Design review of the part built by this model. Coordinates are the model's own, in mm. Round coordinates to 2 decimals unless told otherwise and drop trailing zeros. Loops run counter-clockwise (first coordinate to the right, second up) from the corner with the lowest first, then second, coordinate; pieces in that order, holes last. Notation, with made-up numbers: (12.5, 12.25) - (55.5, 12.25) arc R16 ccw to (55.5, 40.25) - close; hole circle Ø7 at (-34, 20). An arc over 180 degrees is marked (long way). Return JSON: item names as keys, results as strings. Group by question number.
(1) We need section B-B, the plane y = 10.1. Write out the cut boundary in (x, z), and give its area (3 significant figures).
(2) Clearance check with flat-ended pins moving along their axes: pin 1 (0.5 mm diameter, centred on y = 10, z = 35, fed in from -X); pin 2 (0.5 mm diameter, centred on y = 10, z = 56.5, fed in from +X); pin 3 (1.7 mm diameter, centred on x = -9, z = 23.5, fed in from -Y); pin 4 (1.5 mm diameter, centred on x = -11, y = 12, fed in from -Z). State where each tip first meets the part, or that it passes through.
(3) We need section A-A, the plane z = 42. Write out the cut boundary in (x, y), and give its area (3 significant figures).
(4) Wall thickness on L1, parallel to X at y = 12.65, z = 52.5; L2, parallel to Y at x = -9.4, z = 38.5; L3, parallel to Y at x = -11.1, z = 28.5: over which ranges is each line inside the solid? List them lowest first. Write a range as [from, to].
(5) We need section C-C, the plane x = -9.35. Write out the cut boundary in (y, z).
from build123d import *

# Parameters (mm, degrees)
F1_DEPTH = 82.55


with BuildPart() as f1:
    # F0 (on Top) → F1 (new body)
    with BuildSketch(Plane.XY):
        with BuildLine():
            Line((-11.57952, 10.962582), (-11.57952, 9.384583))
            ThreePointArc((-11.57952, 9.384583), (-10.88102, 9.279832), (-10.18252, 9.384583))
            Line((-10.18252, 9.384583), (-10.18252, 10.962582))
            Line((-10.18252, 10.962582), (-8.604521, 10.962582))
            ThreePointArc((-8.604521, 10.962582), (-8.49977, 11.661082), (-8.604521, 12.359582))
            Line((-8.604521, 12.359582), (-10.18252, 12.359582))
            Line((-10.18252, 12.359582), (-10.18252, 13.937582))
            ThreePointArc((-10.18252, 13.937582), (-10.88102, 14.042332), (-11.57952, 13.937582))
            Line((-11.57952, 13.937582), (-11.57952, 12.359582))
            Line((-11.57952, 12.359582), (-13.157519, 12.359582))
            ThreePointArc((-13.157519, 12.359582), (-13.26227, 11.661082), (-13.157519, 10.962582))
            Line((-13.157519, 10.962582), (-11.57952, 10.962582))
        make_face()
    extrude(amount=F1_DEPTH)


solid = f1.part
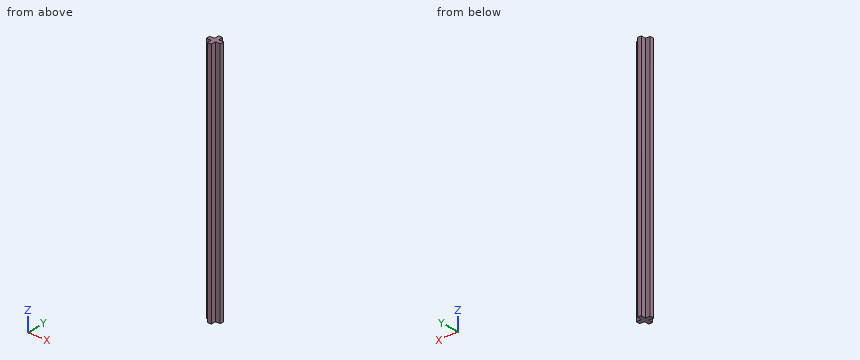
Solutions:
{
 "1": {"outline": "(-11.58, 0) - (-10.18, 0) - (-10.18, 82.55) - (-11.58, 82.55) - close", "area": "115 mm^2"},
 "2": {"pin 1": "x = -11.58", "pin 2": "x = -10.18", "pin 3": "y = 10.96", "pin 4": "z = 0"},
 "3": {"outline": "(-13.16, 10.96) - (-11.58, 10.96) - (-11.58, 9.38) arc R2.38 ccw to (-10.18, 9.38) - (-10.18, 10.96) - (-8.6, 10.96) arc R2.38 ccw to (-8.6, 12.36) - (-10.18, 12.36) - (-10.18, 13.94) arc R2.38 ccw to (-11.58, 13.94) - (-11.58, 12.36) - (-13.16, 12.36) arc R2.38 ccw to start", "area": "11.2 mm^2"},
 "4": {"L1": "[-11.58, -10.18]", "L2": "[10.96, 12.36]", "L3": "[9.29, 14.03]"},
 "5": {"outline": "(10.96, 0) - (12.36, 0) - (12.36, 82.55) - (10.96, 82.55) - close"}
}
